Autodesk Fusion 360 part; units mm, degrees
sketch "Sketch1" plane through (0, 0, 0) normal (0, 1, 0) x (1, 0, 0)
  line L0 (15, 42) -> (15, -58.5)
  line L1 (13, -60.5) -> (-13.5, -60.5)
  line L2 (-15.5, -58.5) -> (-15.5, 53)
  line L3 (-13.5, 55) -> (19, 55)
  line L4 (21, 57) -> (21, 62)
  line L5 (19, 64) -> (-19.9844, 64)
  line L6 (-21.9844, 61.9844) -> (-20.9999, -64.0156)
  line L7 (-19, -66) -> (20, -66)
  line L8 (22, -64) -> (22, 42)
  line L9 (20, 44) -> (17, 44)
  arc A0 (22, 42) -> (20, 44) centre (20, 42) ccw
  arc A1 (17, 44) -> (15, 42) centre (17, 42) ccw
  arc A2 (20, -66) -> (22, -64) centre (20, -64) ccw
  arc A3 (13, -60.5) -> (15, -58.5) centre (13, -58.5) ccw
  arc A4 (-20.9999, -64.0156) -> (-19, -66) centre (-19, -64) ccw
  arc A5 (-15.5, -58.5) -> (-13.5, -60.5) centre (-13.5, -58.5) ccw
  arc A6 (-13.5, 55) -> (-15.5, 53) centre (-13.5, 53) ccw
  arc A7 (19, 55) -> (21, 57) centre (19, 57) ccw
  arc A8 (21, 62) -> (19, 64) centre (19, 62) ccw
  arc A9 (-19.9844, 64) -> (-21.9844, 61.9844) centre (-19.9844, 62) ccw
  dimension "d1" = 2
extrude "Extrude1" add sketch "Sketch1" along normal blind 3.5
sketch "Sketch2" plane through (0, 3.5, 0) normal (0, 1, 0) x (-1, 0, 0)
  line L0 (13.5, -55) -> (-19, -55)
  arc A0 (-19, -55) -> (-21, -57) centre (-19, -57) ccw
  line L1 (-21, -57) -> (-21, -62)
  arc A1 (-21, -62) -> (-19, -64) centre (-19, -62) ccw
  line L2 (-19, -64) -> (19.9844, -64)
  arc A2 (19.9844, -64) -> (21.9844, -61.9844) centre (19.9844, -62) ccw
  line L3 (21.9844, -61.9844) -> (20.9999, 64.0156)
  arc A3 (20.9999, 64.0156) -> (19, 66) centre (19, 64) ccw
  line L4 (19, 66) -> (-20, 66)
  arc A4 (-20, 66) -> (-22, 64) centre (-20, 64) ccw
  line L5 (-22, 64) -> (-22, -42)
  arc A5 (-22, -42) -> (-20, -44) centre (-20, -42) ccw
  line L6 (-20, -44) -> (-17, -44)
  arc A6 (-17, -44) -> (-15, -42) centre (-17, -42) ccw
  line L7 (-15, -42) -> (-15, 58.5)
  arc A7 (-13, 60.5) -> (-15, 58.5) centre (-13, 58.5) ccw
  line L8 (-13, 60.5) -> (13.5, 60.5)
  arc A8 (15.5, 58.5) -> (13.5, 60.5) centre (13.5, 58.5) ccw
  line L9 (15.5, 58.5) -> (15.5, -53)
  arc A9 (13.5, -55) -> (15.5, -53) centre (13.5, -53) ccw
  line L10 (-14.988, 67.5) -> (15.5, 67.5)
  line L11 (15.5, 67.5) -> (15.5, 58.5)
  line L12 (15.5, 58.5) -> (-14.988, 58.5)
  line L13 (-14.988, 58.5) -> (-14.988, 67.5)
sketch "Sketch3" plane through (0, 0, 0) normal (0, -1, 0) x (1, 0, 0)
  line L0 (19, -55) -> (-13.5, -55)
  arc A0 (-15.5, -53) -> (-13.5, -55) centre (-13.5, -53) ccw
  line L1 (-15.5, -53) -> (-15.5, 58.5)
  arc A1 (-13.5, 60.5) -> (-15.5, 58.5) centre (-13.5, 58.5) ccw
  line L2 (-13.5, 60.5) -> (13, 60.5)
  arc A2 (15, 58.5) -> (13, 60.5) centre (13, 58.5) ccw
  line L3 (15, 58.5) -> (15, -42)
  arc A3 (15, -42) -> (17, -44) centre (17, -42) ccw
  line L4 (17, -44) -> (20, -44)
  arc A4 (20, -44) -> (22, -42) centre (20, -42) ccw
  line L5 (22, -42) -> (22, 64)
  arc A5 (22, 64) -> (20, 66) centre (20, 64) ccw
  line L6 (20, 66) -> (-19, 66)
  arc A6 (-19, 66) -> (-20.9999, 64.0156) centre (-19, 64) ccw
  line L7 (-20.9999, 64.0156) -> (-21.9844, -61.9844)
  arc A7 (-21.9844, -61.9844) -> (-19.9844, -64) centre (-19.9844, -62) ccw
  line L8 (-19.9844, -64) -> (19, -64)
  arc A8 (19, -64) -> (21, -62) centre (19, -62) ccw
  line L9 (21, -62) -> (21, -57)
  arc A9 (21, -57) -> (19, -55) centre (19, -57) ccw
  line L10 (-15.5, 51.9243) -> (14.988, 51.9243)
  line L11 (14.988, 51.9243) -> (14.988, 76)
  line L12 (14.988, 76) -> (-15.5, 76)
  line L13 (-15.5, 76) -> (-15.5, 51.9243)
extrude "Extrude3" cut sketch "Sketch3" against normal blind 1.5 contours A1 L2 A2 L6 L11 L13
sketch "Sketch4" plane through (0, 3.5, 0) normal (0, 1, 0) x (-1, 0, 0)
  line L0 (13.5, -55) -> (-19, -55)
  arc A0 (-19, -55) -> (-21, -57) centre (-19, -57) ccw
  line L1 (-21, -57) -> (-21, -62)
  arc A1 (-21, -62) -> (-19, -64) centre (-19, -62) ccw
  line L2 (-19, -64) -> (19.9844, -64)
  arc A2 (19.9844, -64) -> (21.9844, -61.9844) centre (19.9844, -62) ccw
  line L3 (21.9844, -61.9844) -> (20.9999, 64.0156)
  arc A3 (20.9999, 64.0156) -> (19, 66) centre (19, 64) ccw
  line L4 (19, 66) -> (-20, 66)
  arc A4 (-20, 66) -> (-22, 64) centre (-20, 64) ccw
  line L5 (-22, 64) -> (-22, -42)
  arc A5 (-22, -42) -> (-20, -44) centre (-20, -42) ccw
  line L6 (-20, -44) -> (-17, -44)
  arc A6 (-17, -44) -> (-15, -42) centre (-17, -42) ccw
  line L7 (-15, -42) -> (-15, 58.5)
  arc A7 (-13, 60.5) -> (-15, 58.5) centre (-13, 58.5) ccw
  line L8 (-13, 60.5) -> (13.5, 60.5)
  arc A8 (15.5, 58.5) -> (13.5, 60.5) centre (13.5, 58.5) ccw
  line L9 (15.5, 58.5) -> (15.5, -53)
  arc A9 (13.5, -55) -> (15.5, -53) centre (13.5, -53) ccw
  line L10 (-15, -24.5) -> (17.4682, -24.5)
  line L11 (17.4682, -24.5) -> (17.4682, -18)
  line L12 (17.4682, -18) -> (-15, -18)
  line L13 (-15, -18) -> (-15, -24.5)
  line L14 (-15, 16.5) -> (17, 16.5)
  line L15 (17, 16.5) -> (17, 22.5)
  line L16 (17, 22.5) -> (-15, 22.5)
  line L17 (-15, 22.5) -> (-15, 16.5)
  line L18 (-13, 60.5) -> (13.5, 60.5)
  line L19 (-16.3717, -55) -> (5.5, -55)
  line L20 (5.5, -55) -> (5.5, -64)
  line L21 (5.5, -64) -> (-16.3717, -64)
  line L22 (-16.3717, -64) -> (-16.3717, -55)
  dimension "d10" = 6.5
  dimension "d11" = 6
  dimension "d12" = 38
  dimension "d13" = 78.5
extrude "Extrude4" add sketch "Sketch4" against normal blind 1 contours L7 L9 L10 L12 L13 | L7 L9 L14 L16 L17
sketch "Sketch5" plane through (0, 0, 0) normal (0, -1, 0) x (1, 0, 0)
  line L0 (-15.5, -53) -> (-15.5, 66)
  line L1 (-15.5, 66) -> (-19, 66)
  arc A0 (-19, 66) -> (-20.9999, 64.0156) centre (-19, 64) ccw
  line L2 (-20.9999, 64.0156) -> (-21.9844, -61.9844)
  arc A1 (-21.9844, -61.9844) -> (-19.9844, -64) centre (-19.9844, -62) ccw
  line L3 (-19.9844, -64) -> (19, -64)
  arc A2 (19, -64) -> (21, -62) centre (19, -62) ccw
  line L4 (21, -62) -> (21, -57)
  arc A3 (21, -57) -> (19, -55) centre (19, -57) ccw
  line L5 (19, -55) -> (-13.5, -55)
  arc A4 (-15.5, -53) -> (-13.5, -55) centre (-13.5, -53) ccw
  line L6 (16.5, -64) -> (-5, -64)
  line L7 (-5, -64) -> (-5, -55)
  line L8 (-5, -55) -> (16.5, -55)
  line L9 (16.5, -55) -> (16.5, -64)
extrude "Extrude5" cut sketch "Sketch5" against normal blind 2 contours L3 L5 L6 L7 L8 L9
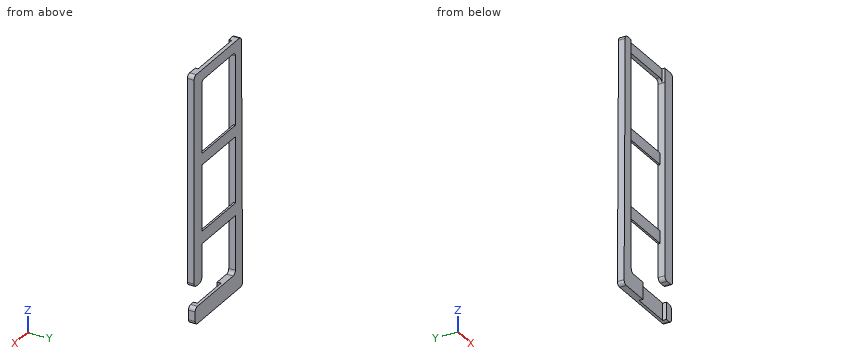
Model file for the job. Use its own axes, mm. Give positions to 0.01 mm unless a question says otherwise; leave off trailing zeros. Order: outer loops, then holes, each group sorted by start corner. A loop starts at its lowest first (then second) coordinate and runs counter-clockwise, first axis right, second up. Notation, with made-up numbers: M -16.75,-2 L -1.75,-2 A9 cw -1.75,11 Z; hole C 37,-27 d6. An arc over 180 degrees is marked long. Put each result on its own line as item: value. Start each with the question number.
(1) Band-saw the part on B-B on x = -8. Give the cut face in (y, z), then the cut area to 3 significant figures.
(2) Drill centre lines: L1, parallel to Z at x = 18.5, y = 1.35; L2, parallel to Z at x = 8.5, y = 3.05; L3, parallel to Z at x = 6, y = 2.1. Where is each one in solid material? Low to high. Write a range as [from, to].
(3) Band-saw the part on C-C on z = 45. Give the cut face in (x, y).
(4) Pin check, flat tips, straight feed: pin 1 Ø1.2 at (y, z) = (0.5, 61.5) entering from -X; pin 2 Ø7 at (x, z) = (-2, -22) entering from -Y; pin 3 Ø1 at (y, z) = (1.5, -57.5) entering from -X; pin 4 Ø8 at (x, z) = (-9, -2) entering from -Y. Stop position of each tip, or through.
(5) Band-saw the part on A-A on y = 0.95. Give the cut face in (x, z).
(6) Band-saw the part on D-D on x = -2. Give the cut face in (y, z), then the cut area to 3 significant figures.
Results below:
1. outline: M 0,-64 L 3.5,-64 L 3.5,-55 L 0,-55 Z; M 1.5,60.5 L 3.5,60.5 L 3.5,66 L 1.5,66 Z; M 2.5,-24.5 L 3.5,-24.5 L 3.5,-18 L 2.5,-18 Z; M 2.5,16.5 L 3.5,16.5 L 3.5,22.5 L 2.5,22.5 Z
1. area: 55.0 mm2
2. L1: z = [-64, -55], [-44, 66]
2. L2: z = [-64, -55], [-24.5, -18], [16.5, 22.5], [60.5, 66]
2. L3: z = [-64, -55], [60.5, 66]
3. outline: M -21.15,0 L -15.5,0 L -15.5,3.5 L -21.15,3.5 Z; M 15,0 L 22,0 L 22,3.5 L 15,3.5 Z
4. pin 1: stops at x = -21.02
4. pin 2: stops at y = 2.5
4. pin 3: stops at x = -21.95
4. pin 4: passes through
5. outline: M -21.98,-61.98 A2 ccw -19.98,-64 L -5,-64 L -5,-55 L -13.5,-55 A2 cw -15.5,-53 L -15.5,66 L -19,66 A2 ccw -21,64.02 Z; M 14.99,58.72 A2 cw 15,58.5 L 15,-42 A2 ccw 17,-44 L 20,-44 A2 ccw 22,-42 L 22,64 A2 ccw 20,66 L 14.99,66 Z; M 16.5,-64 L 19,-64 A2 ccw 21,-62 L 21,-57 A2 ccw 19,-55 L 16.5,-55 Z
6. outline: M 1.5,60.5 L 3.5,60.5 L 3.5,66 L 1.5,66 Z; M 2,-64 L 3.5,-64 L 3.5,-55 L 2,-55 Z; M 2.5,-24.5 L 3.5,-24.5 L 3.5,-18 L 2.5,-18 Z; M 2.5,16.5 L 3.5,16.5 L 3.5,22.5 L 2.5,22.5 Z
6. area: 37.0 mm2
